Part model, mm, in its own coordinate system. A direction names the side the tool comes from. Round coordinates to 2 decimals unless told otherwise and drop trailing zeros. Order: outer loops, then holes, each group sorted by start corner. A loop starts at its lowest first (then second) coordinate and runs counter-clockwise, first axis right, second up. Notation, with made-up numbers: (10.25, 68.5) -> (16.25, 68.5) arc R11 cw to (16.25, 81.5) -> close; hole circle Ø6 at (-37, 41). An arc over 180 degrees is marked (long way). Use CSV: the item, a comma, the result in double quotes.
```python
from build123d import *

# Parameters (mm, degrees)
SKETCH1_R               = 2
BOSS_EXTRUDE1_DEPTH     = 10
SKETCH6_R               = 7.5
BOSS_EXTRUDE3_DEPTH     = 5
CUT_EXTRUDE4_DEPTH      = 26.013853674
CUT_EXTRUDE4_DEPTH_BACK = 26.013853674
SKETCH7_R               = 2
SKETCH10_R              = 7.5
CUT_EXTRUDE7_DEPTH      = 9
SKETCH11_W              = 4
SKETCH11_H              = 4
BOSS_EXTRUDE4_DEPTH     = 2.5
FILLET1_R               = 2
SKETCH12_R              = 0.5
CUT_EXTRUDE8_DEPTH      = 10


with BuildPart() as part:
    # Sketch1 → Boss-Extrude1 (new body)
    with BuildSketch(Plane.XY):
        with BuildLine():
            Line((5.026455026, -10.023549892), (-4.973544974, -10.023549892))
            Line((-4.973544974, -10.023549892), (-4.973544974, 4.386280164))
            ThreePointArc((-4.973544974, 4.386280164), (0.026455026, 17.476450108), (5.026455026, 4.386280164))
            Line((5.026455026, 4.386280164), (5.026455026, -10.023549892))
        make_face()
        with Locations((0.026455026, 9.976450108)):
            Circle(SKETCH1_R, mode=Mode.SUBTRACT)
    extrude(amount=BOSS_EXTRUDE1_DEPTH)

    # Sketch6 → Boss-Extrude3 (add, symmetric)
    with BuildSketch(Plane(origin=(2.513227513, 0, 2.513227513), x_dir=(-0.7071067811865477, 0, 0.7071067811865475), z_dir=(-0.7071067811865475, 0, -0.7071067811865477))):
        with Locations((3.516827377, -10.023549892)):
            Circle(SKETCH6_R)
    extrude(amount=BOSS_EXTRUDE3_DEPTH, both=True)

    # Sketch7 → Cut-Extrude4 (cut, two sides: drawn at the far end of the back side and taken through both)
    with BuildSketch(Plane(origin=(-1.022306393, 0, -1.022306393), x_dir=(-0.7071067811865476, 0, 0.7071067811865476), z_dir=(-0.7071067811865476, 0, -0.7071067811865476)).offset(-CUT_EXTRUDE4_DEPTH_BACK)):
        with Locations((3.516827377, -10.023549892)):
            Circle(SKETCH7_R)
    extrude(amount=CUT_EXTRUDE4_DEPTH + CUT_EXTRUDE4_DEPTH_BACK, mode=Mode.SUBTRACT)

    # Sketch10 → Cut-Extrude7 (cut)
    with BuildSketch(Plane(origin=(6.048761419, 0, 6.048761419), x_dir=(0.7071067811865476, 0, -0.7071067811865476), z_dir=(0.7071067811865476, 0, 0.7071067811865476))):
        with Locations((-3.516827377, -10.023549892)):
            Circle(SKETCH10_R)
    cut_extrude7 = extrude(amount=CUT_EXTRUDE7_DEPTH, mode=Mode.SUBTRACT)

    # Mirror1: Cut-Extrude7 across plane
    add(cut_extrude7.mirror(Plane(origin=(2.513227513, 0, 2.513227513), x_dir=(-0.7071067811865478, 0, 0.7071067811865472), z_dir=(-0.7071067811865475, 0, -0.7071067811865477))), mode=Mode.SUBTRACT)

    # Sketch11 → Boss-Extrude4 (add, symmetric)
    with BuildSketch(Plane(origin=(0, -17.5, 0), x_dir=(1, 0, 0), z_dir=(0, 1, 0))):
        with Locations((0.026455026, -5)):
            Rectangle(SKETCH11_W, SKETCH11_H)
    extrude(amount=BOSS_EXTRUDE4_DEPTH, both=True)

    # Fillet1
    # the kernel refuses this fillet: 2 mm, written as the material it adds along each edge
    with BuildSketch(Plane(origin=(3.561988932, -10.023549892, 8.535533906), x_dir=(0.5737197168089216, 0.5845437306903406, -0.5737197168089216), z_dir=(0.4133348358712229, -0.8113622045120283, -0.4133348358712229))) as fillet1_piece_1_section:
        with BuildLine():
            CenterArc((7.5 - FILLET1_R, FILLET1_R), FILLET1_R, 270, 90)
            Line((7.5 - FILLET1_R, 0), (7.5, 0))
            Line((7.5, 0), (7.5, FILLET1_R))
        make_face()
    fillet1_piece_1 = revolve(axis=Axis((3.561988932, -10.023549892, 8.535533906), (0.7071067811865476, 0, 0.7071067811865476)), revolution_arc=108.458473571, mode=Mode.PRIVATE)
    fillet1_piece_1 = split(fillet1_piece_1, bisect_by=Plane(origin=(5.026455026, -3.097280079, 8.789305728), z_dir=(-1, 0, 0)), keep=Keep.TOP, mode=Mode.PRIVATE)
    fillet1_piece_1 = split(fillet1_piece_1, bisect_by=Plane(origin=(3.815760609, -3.097280079, 10), z_dir=(0, 0, -1)), keep=Keep.TOP, mode=Mode.PRIVATE)
    add(fillet1_piece_1)
    with BuildSketch(Plane(origin=(-3.509078879, -10.023549892, 1.464466094), x_dir=(0.5737197168089216, 0.584543730690341, -0.5737197168089213), z_dir=(0.4133348358712232, -0.8113622045120281, -0.4133348358712231))) as fillet1_piece_2_section:
        with BuildLine():
            CenterArc((7.5 - FILLET1_R, -FILLET1_R), FILLET1_R, 0, 90)
            Line((7.5 - FILLET1_R, 0), (7.5, 0))
            Line((7.5, 0), (7.5, -FILLET1_R))
        make_face()
    fillet1_piece_2 = revolve(axis=Axis((-3.509078879, -10.023549892, 1.464466094), (0.7071067811865475, 0, 0.7071067811865477)), revolution_arc=108.458473571, mode=Mode.PRIVATE)
    fillet1_piece_2 = split(fillet1_piece_2, bisect_by=Plane(origin=(-3.762850661, -3.097280076, 0), z_dir=(0, 0, 1)), keep=Keep.TOP, mode=Mode.PRIVATE)
    fillet1_piece_2 = split(fillet1_piece_2, bisect_by=Plane(origin=(-4.973544974, -3.097280076, 1.21069445), z_dir=(1, 0, 0)), keep=Keep.TOP, mode=Mode.PRIVATE)
    add(fillet1_piece_2)

    # Sketch12 → Cut-Extrude8 (cut)
    with BuildSketch(Plane(origin=(0, 0, 3), x_dir=(-1, 0, 0), z_dir=(0, 0, -1))):
        with Locations((-0.026455026, -18)):
            Circle(SKETCH12_R)
    extrude(amount=-CUT_EXTRUDE8_DEPTH, mode=Mode.SUBTRACT)


solid = part.part
```
(1) Drop flat-ended pins along their axis: P1, Ø1, axis at x = -2.5, y = -7.5, coming from the +Z side; P2, Ø10, axis at y = -11, z = 0, coming from the +X side; P3, Ø2, axis at y = -8.5, z = -2, coming from the +X side; P4, Ø1.5, axis at x = -2.5, y = -9, coming from the +Z side. Give the stop position or say it passes through.
Reply:
P1,"z = 13.02"
P2,"x = 8.87"
P3,"x = 4.45"
P4,"z = 13.74"
(2) Cut at B-B, the plane x = 1.25. State how many separate pieces and enclosed holes the cut face has, then the cut area to 3 significant figures.
Reply:
separate pieces,"2"
enclosed holes,"1"
area,"351 mm2"
(3) Which spindle directions (+Z, -Z, +X, -X, +Y, -Y) get a long thin tool onto all of the face, cutting with end or side? Do faces 1 (the face through (-4.613, -11.701, 2.569)), 2 (the face through (2.5, -11.7, 9.6)), 3 (the face through (-0.227, 17.472, 4.93)). Say none if no direction does.
Reply:
face 1,"-Z, -X, -Y"
face 2,"+Z, +X, -Y"
face 3,"+Z, -Z"
(4) Cut at C-C, the plane y = -0.5. Give the cut face in (x, z).
Reply:
outline,"(-4.97, 0) -> (5.03, 0) -> (5.03, 10) -> (-4.97, 10) -> close"
(5) Cut at A-A, the plane y = -18. Give the cut face in (x, z), then the cut area to 3 significant figures.
Reply:
outline,"(-1.97, 3) -> (-0.47, 3) -> (-0.47, 7) -> (-1.97, 7) -> close; (0.53, 3) -> (2.03, 3) -> (2.03, 7) -> (0.53, 7) -> close"
area,"12.0 mm2"
(6) Probe probe 1 along Z at (x, y) = (-6.25, 12.5); probe 2 along X at (y, z) = (8.5, 1.75); probe 3 along Y at (x, z) = (4.25, 7.25). List the from-to ranges inside material, lowest first. Write a range as [from, to].
Reply:
probe 1,"[0, 10]"
probe 2,"[-7.33, -1.32], [1.38, 7.38]"
probe 3,"[-17.39, -11.46], [-8.59, 16.17]"
(7) Pull direction X, two halves, no side cores. Call faces 4 (the face through (-0.23, 11.96, 4.93)), 5 (the face through (2, 8, 0)), 6 (the face through (5.026, 0, 5)): released by +X, released by -X, zero draft, split by the parting line, or undercut.
Reply:
face 4,"undercut"
face 5,"zero draft"
face 6,"released by +X"
